from build123d import *

# Parameters (mm, degrees)
F1_W     = 61.55309
F1_H     = 58.615133
F2_DEPTH = 25.4
F3_W     = 61.55309
F3_H     = 12.171417
F4_DEPTH = 25.4


with BuildPart() as f2:
    # F1 (on offset) → F2 (new body)
    with BuildSketch(Plane.XZ.offset(25.4)):
        with Locations((45.909398, 46.550103)):
            Rectangle(F1_W, F1_H)
    extrude(amount=F2_DEPTH)

    # F3 (on face) → F4 (join)
    with BuildSketch(Plane.XZ.offset(50.8)):
        with Locations((45.909398, 69.771961)):
            Rectangle(F3_W, F3_H)
    extrude(amount=F4_DEPTH)


solid = f2.part
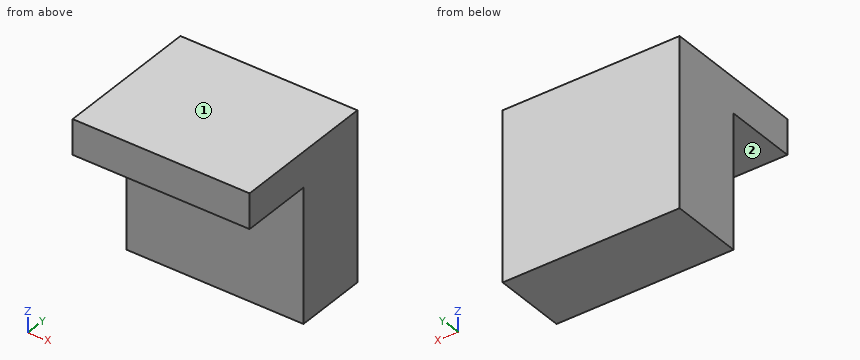
Part model, mm, in its own coordinate system. Face numbers are marked on the shaded views. A direction names the side the tool comes from. Give positions to 0.01 mm unless a question says otherwise; leave off trailing zeros. Loops run counter-clockwise (first coordinate to the right, second up) from the corner with the lowest first, then second, coordinate; pieces in that order, holes last. Notation, with made-up numbers: (56.5, 84) -> (102.5, 84) arc R10 ccw to (102.5, 101) -> close; hole circle Ø11 at (-33.75, 20.5). An arc over 180 degrees is marked (long way). Write each question's results on one line, items separated by ' | '. Start each with the question number.
Q1. Pin check, flat tips, straight feed: P1, Ø8, axis at x = 45, z = 43, coming from the -Y side; P2, Ø6, axis at x = 54, y = -60, coming from the -Z side. Stop position of each tip, or through.
Q2. Which spindle directions (+Z, -Z, +X, -X, +Y, -Y) get a long thin tool onto all of the face, cutting with end or side? Do the marked faces 1 and 2. Say none if no direction does.
Q3. Wall check: L1, parallel to Y at x = 29.5, z = 57.5; L2, parallel to Z at x = 20, y = -59. Give the ranges that are in metal, low to high.
Q4. Band-saw the part on C-C on z = 60. List the corners of the cut face in (x, y).
Q5. Band-saw the part on B-B on y = -62.5. List the corners of the cut face in (x, z).
Q6. Band-saw the part on A-A on x = 73. List the corners of the cut face in (y, z), plus the area to 3 significant figures.
Results are:
1) P1: stops at y = -50.8 | P2: stops at z = 63.69
2) face 1: +Z, +X, -X, +Y, -Y | face 2: -Z, +X, -X, -Y
3) L1: y = -50.8 to -25.4 | L2: z = 63.69 to 75.86
4) outline: (15.13, -50.8) -> (76.69, -50.8) -> (76.69, -25.4) -> (15.13, -25.4) -> close
5) outline: (15.13, 63.69) -> (76.69, 63.69) -> (76.69, 75.86) -> (15.13, 75.86) -> close
6) outline: (-76.2, 63.69) -> (-50.8, 63.69) -> (-50.8, 17.24) -> (-25.4, 17.24) -> (-25.4, 75.86) -> (-76.2, 75.86) -> close | area: 1,800 mm²
